CAD build for the part. Positions are in the model's coordinates, mm. A direction names the side the tool comes from. Give positions to 0.01 mm unless a question says otherwise; leave off trailing zeros. Write each loop counter-clockwise with the first axis right and the second up, starting at its lowest first coordinate (ties: lowest second). Pieces come first, ordered by that corner, then holes. Notation, with made-up numbers: (73, 80.5) -> (98, 80.5) arc R28 cw to (98, 117.5) -> close; hole circle Ø10 at (63.25, 68.5). An arc over 180 degrees is marked (long way). Answer as a JSON object with one key per item and string values.
```python
from build123d import *

# Parameters (mm, degrees)
SKETCH8_R               = 2.15
BOSS_EXTRUDE2_DEPTH     = 7
SKETCH9_R               = 1.975
CUT_EXTRUDE5_DEPTH      = 10
CUT_EXTRUDE6_DEPTH      = 10
CUT_EXTRUDE6_DEPTH_BACK = 10
CHAMFER1_SIZE           = 1.5


with BuildPart() as part:
    # Sketch8 → Boss-Extrude2 (new body)
    with BuildSketch(Plane(origin=(0, 0, 0), x_dir=(1, 0, 0), z_dir=(0, 1, 0))):
        with BuildLine():
            Line((0, -4), (0, 4))
            Line((0, 4), (19.848380493, 4.647527464))
            ThreePointArc((19.848380493, 4.647527464), (24.65, 0), (19.848380493, -4.647527464))
            Line((19.848380493, -4.647527464), (0, -4))
        make_face()
        with Locations(Location((20, 0, 0), (0, 0, 270))):
            Circle(SKETCH8_R, mode=Mode.SUBTRACT)
    extrude(amount=BOSS_EXTRUDE2_DEPTH)

    # Sketch9 → Cut-Extrude5 (cut)
    with BuildSketch(Plane.ZY):
        with Locations((0, 3.5)):
            Circle(SKETCH9_R)
    extrude(amount=-CUT_EXTRUDE5_DEPTH, mode=Mode.SUBTRACT)

    # Sketch10 → Cut-Extrude6 (cut, two sides: drawn at the far end of the back side and taken through both)
    with BuildSketch(Plane.XY.offset(-CUT_EXTRUDE6_DEPTH_BACK)):
        Polygon((9.924190246, 7), (15.408042822, 3), (24.65, 3), (24.65, 7), align=None)
    extrude(amount=CUT_EXTRUDE6_DEPTH + CUT_EXTRUDE6_DEPTH_BACK, mode=Mode.SUBTRACT)

    # Chamfer1
    chamfer1_edges = [part.edges().sort_by_distance(p)[0] for p in [
        (4.962095123, 7, 4.161881866),
        (4.962095123, 7, -4.161881866),
        (9.924190246, 0, -4.323763732),
        (24.65, 0, 0),
        (9.924190246, 0, 4.323763732),
    ]]
    chamfer(chamfer1_edges, length=CHAMFER1_SIZE)


solid = part.part
```
1) Wall check: probe 1 along X at (y, z) = (2.35, 0); probe 2 along Y at (x, z) = (6.25, 0) (3 decimals); probe 3 along X at (y, z) = (1.35, 0). Give the ranges that are in metal, low to high.
Model answer:
{"probe 1": "x = 10 to 17.85, 22.15 to 24.65", "probe 2": "y = 0 to 1.525, 5.475 to 7", "probe 3": "x = 0 to 17.85, 22.15 to 24.5"}
2) Slice it at A-A (z = 0). List the corners of the cut face in (x, y) (3 decimals).
Model answer:
{"outline": "(0, 0) -> (17.85, 0) -> (17.85, 3) -> (15.408, 3) -> (9.924, 7) -> (0, 7) -> (0, 5.475) -> (10, 5.475) -> (10, 1.525) -> (0, 1.525) -> close; (22.15, 0) -> (23.15, 0) -> (24.65, 1.5) -> (24.65, 3) -> (22.15, 3) -> close"}
3) Mould opens along Z. For faces 4 (the conical face through (23.39, 0.24, -0.08)), 5 (the flat face through (12.628, 5.028, -0.063)), 6 (the cylindrical face through (17.9, 1.48, -0.47)) say: released by +Z, released by -Z, zero draft, split by the parting line, or undercut.
Model answer:
{"face 4": "split by the parting line", "face 5": "zero draft", "face 6": "undercut"}
4) Slice it at B-B (x = 5.75). List the corners of the cut face in (y, z) (3 decimals), then the cut area to 3 significant figures.
Model answer:
{"outline": "(0, -2.687) -> (1.5, -4.188) -> (5.5, -4.188) -> (7, -2.687) -> (7, 2.687) -> (5.5, 4.188) -> (1.5, 4.188) -> (0, 2.687) -> close; hole circle Ø3.95 at (3.5, 0)", "area": "41.9 mm2"}
5) Slice it at D-D (x = 16). List the corners of the cut face in (y, z), then the cut area to 3 significant figures.
Model answer:
{"outline": "(0, -3.02) -> (1.5, -4.52) -> (3, -4.52) -> (3, 4.52) -> (1.5, 4.52) -> (0, 3.02) -> close", "area": "24.9 mm2"}
6) 3-axis set-ups, long thin cutter, end or side, ignore diameter. For faces 1 (the flat face through (10, 4, 0)), 2 (the flat face through (0, 1, 0)), 3 (the flat face through (17.9, 3, 1)): which of +Z, -Z, +X, -X, +Y, -Y reach the whole face in a straight line?
Model answer:
{"face 1": "-X", "face 2": "+Z, -Z, -X, +Y, -Y", "face 3": "+Z, -Z, +X, +Y"}
7) Pin check, flat tip, straight feed: pin 1 (5.5 mm diameter, centred on x = 20, z = 0, fed in from +Y). Stop position of the tip, or through.
Model answer:
{"pin 1": "stops at y = 3"}
8) Slice it at C-C (y = 3.5). List the corners of the cut face in (x, z) (3 decimals), then the cut area to 3 significant figures.
Model answer:
{"outline": "(0, -4) -> (14.723, -4.48) -> (14.723, 4.48) -> (0, 4) -> (0, 1.975) -> (10, 1.975) -> (10, -1.975) -> (0, -1.975) -> close", "area": "85.4 mm2"}
